Geometry: final body of the model. Coordinates: model frame, mm. Face numbers are marked on the shaded views. A direction names the side the tool comes from. Give positions to 0.01 mm unless a question says otherwise; leave off trailing zeros. Write each loop counter-clockwise with the first axis right and the second up, starting at its lowest first coordinate (ties: lowest second). Pieces come first, ordered by that corner, then holes. Notation, with made-up numbers: (24.5, -30.5) -> (67.5, -30.5) arc R17 cw to (67.5, -14.5) -> close; hole circle Ø9 at (36, 24). An arc over 180 degrees is marked (long way). Answer in a Markdown table with one row per item. Add a question column.
Item 1: Access query for the marked faces 4, 5 and 6. Directions: +Z, -Z, +X, -X, +Y, -Y. A direction counts if a zero-diameter tool reaches every point of the face in a straight line with its end or side. Return the directions, or none.
Item 2: Section query B-B on y = 24.75. Output: boundary loops of the cut face in (x, z).
Item 3: Section query A-A on z = 12.7. Output: boundary loops of the cut face in (x, y), plus the area to 3 significant figures.
Item 4: Draft query along Z for the marked faces 1, 2 and 3. Return one class per face: +Z half, -Z half, draft (parallel to the pull), parting line (faces both ways), or undercut.
Item 5: Section query C-C on x = 1.75. Output: boundary loops of the cut face in (y, z), plus the area to 3 significant figures.
Item 6: Section query D-D on x = 8.5. Output: boundary loops of the cut face in (y, z).
Item 7: Material intervals for probe 1 along Y at (x, z) = (-1.5, 21.25); probe 2 along Y at (x, z) = (0.75, 19.5); probe 3 along Z at (x, y) = (5.25, 21.25), sorted ascending. Write a range as from..to.
Item 8: First-contact query: P1, Ø2, axis at x = 12, y = 21.5, coming from the -Z side; P2, Ø1.5, axis at x = -4.5, z = 13, coming from the -Y side; P3, Ø8, axis at y = 33, z = 12.5, coming from the +X side. Flat tips, straight axial feed; report the tip coordinate or a pass-through.
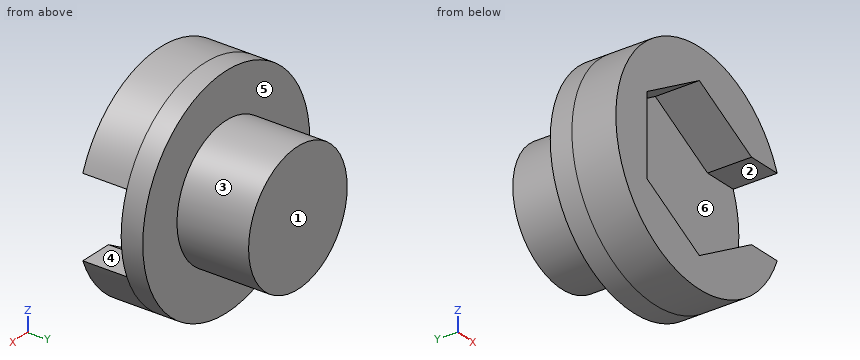
```python
from build123d import *

# Parameters (mm, degrees)
BOSS_EXTRUDE1_DEPTH = 25.4
BOSS_EXTRUDE3_DEPTH = 5.08
SKETCH4_W           = 37.4
SKETCH4_H           = 25.4
CUT_EXTRUDE1_DEPTH  = 25.4
SKETCH5_R           = 12.7
BOSS_EXTRUDE4_DEPTH = 2.5
SKETCH6_R           = 7.5
BOSS_EXTRUDE5_DEPTH = 8.272


with BuildPart() as part:
    # Sketch1 → Boss-Extrude1 (new body)
    with BuildSketch(Plane.XY):
        Polygon((-10.189534884, 0), (-10.189534884, 9), (15.210465116, 9), (15.210465116, 0), (21.210465116, 0), (21.210465116, 20.17346), (-16.189534884, 20.17346), (-16.189534884, 0), align=None)
    extrude(amount=BOSS_EXTRUDE1_DEPTH)

    # Sketch3 → Boss-Extrude3 (add)
    with BuildSketch(Plane(origin=(0, 20.17346, 0), x_dir=(1, 0, 0), z_dir=(0, 1, 0))):
        with BuildLine():
            Line((14.354818113, -17.282717762), (10.447965116, -17.282717762))
            Line((10.447965116, -17.282717762), (2.510465116, -21.865435523))
            Line((2.510465116, -21.865435523), (-5.427034884, -17.282717762))
            Line((-5.427034884, -17.282717762), (-5.427034884, -8.117282238))
            Line((-5.427034884, -8.117282238), (2.510465116, -3.534564477))
            Line((2.510465116, -3.534564477), (10.447965116, -8.117282238))
            Line((10.447965116, -8.117282238), (14.354818113, -8.117282238))
            ThreePointArc((14.354818113, -8.117282238), (-10.189534884, -12.7), (14.354818113, -17.282717762))
        make_face()
    extrude(amount=BOSS_EXTRUDE3_DEPTH)

    # Sketch4 → Cut-Extrude1 (cut)
    with BuildSketch(Plane(origin=(0, 20.17346, 0), x_dir=(1, 0, 0), z_dir=(0, 1, 0))):
        with Locations((2.510465116, -12.7)):
            Rectangle(SKETCH4_W, SKETCH4_H)
    extrude(amount=-CUT_EXTRUDE1_DEPTH, mode=Mode.SUBTRACT)

    # Sketch5 → Boss-Extrude4 (add)
    with BuildSketch(Plane(origin=(0, 25.25346, 0), x_dir=(1, 0, 0), z_dir=(0, 1, 0))):
        with Locations((2.510465116, -12.7)):
            Circle(SKETCH5_R)
    extrude(amount=BOSS_EXTRUDE4_DEPTH)

    # Sketch6 → Boss-Extrude5 (add)
    with BuildSketch(Plane(origin=(0, 27.75346, 0), x_dir=(1, 0, 0), z_dir=(0, 1, 0))):
        with Locations((2.510465116, -12.7)):
            Circle(SKETCH6_R)
    extrude(amount=BOSS_EXTRUDE5_DEPTH)


solid = part.part
```
Findings below:
| question | item | result |
|---|---|---|
| 1 | face 4 | +X, -Y |
| 1 | face 5 | +Y |
| 1 | face 6 | -Y |
| 2 | outline | (-5.43, 8.12) -> (-5.43, 17.28) -> (2.51, 21.87) -> (10.45, 17.28) -> (14.35, 17.28) arc R12.7 ccw (long way) to (14.35, 8.12) -> (10.45, 8.12) -> (2.51, 3.53) -> close |
| 3 | outline | (-10.19, 20.17) -> (-5.43, 20.17) -> (-5.43, 25.25) -> (15.21, 25.25) -> (15.21, 27.75) -> (10.01, 27.75) -> (10.01, 36.03) -> (-4.99, 36.03) -> (-4.99, 27.75) -> (-10.19, 27.75) -> close |
| 3 | area | 212 mm^2 |
| 4 | face 1 | draft |
| 4 | face 2 | undercut |
| 4 | face 3 | parting line |
| 5 | outline | (20.17, 0.02) -> (27.75, 0.02) -> (27.75, 5.24) -> (36.03, 5.24) -> (36.03, 20.16) -> (27.75, 20.16) -> (27.75, 25.38) -> (20.17, 25.38) -> (20.17, 21.43) -> (25.25, 21.43) -> (25.25, 3.97) -> (20.17, 3.97) -> close |
| 5 | area | 227 mm^2 |
| 6 | outline | (20.17, 1.5) -> (27.75, 1.5) -> (27.75, 8.19) -> (36.03, 8.19) -> (36.03, 17.21) -> (27.75, 17.21) -> (27.75, 23.9) -> (20.17, 23.9) -> (20.17, 18.41) -> (25.25, 18.41) -> (25.25, 6.99) -> (20.17, 6.99) -> close |
| 7 | probe 1 | y = 20.17..27.75 |
| 7 | probe 2 | y = 25.25..36.03 |
| 7 | probe 3 | z = 0.3..5.12, 20.28..25.1 |
| 8 | P1 | stops at z = 3.25 |
| 8 | P2 | stops at y = 25.25 |
| 8 | P3 | stops at x = 10.01 |
